Input: dimensioned drawing with shaded views. Units: mm. Origin: part minimum x, y, z. Coordinates: 2 decimals unless noted, no trailing zeros. Loops run counter-clockwise (first coordinate to the right, second up) from the corner with the lowest first, then second, coordinate; pieces in that order, holes last.
(1) Section C-C, the plane x = 20. Return loops of the section in (y, z), then the cut area to 3 significant figures.
(2) Section B-B, the plane z = 6. Return loops of the section in (x, y), then the cut area to 3 significant figures.
(3) Section A-A, the plane y = 8. Return loops of the section in (x, z), then the cut area to 3 significant figures.
(4) Contact query for a flat-ended pin moving along its axis: P1, Ø1.5, axis at x = 35.5, z = 6, coming from the -Y side. Output: stop coordinate, or through.
(5) Line query: L1, parallel to X at y = 2.25, z = 6; L2, parallel to Y at x = 20, z = 11.25; L3, parallel to X at y = 4, z = 4.75. Output: solid intervals per line, ascending.
(6) Section D-D, the plane y = 1.5. Return loops of the section in (x, z), then the cut area to 3 significant figures.
(7) Mould query, pull axis X, two halves, no side actions, for the marked faces 1, 2 and 3. Classes: released by +X, released by -X, zero draft, split by the parting line, or undercut.
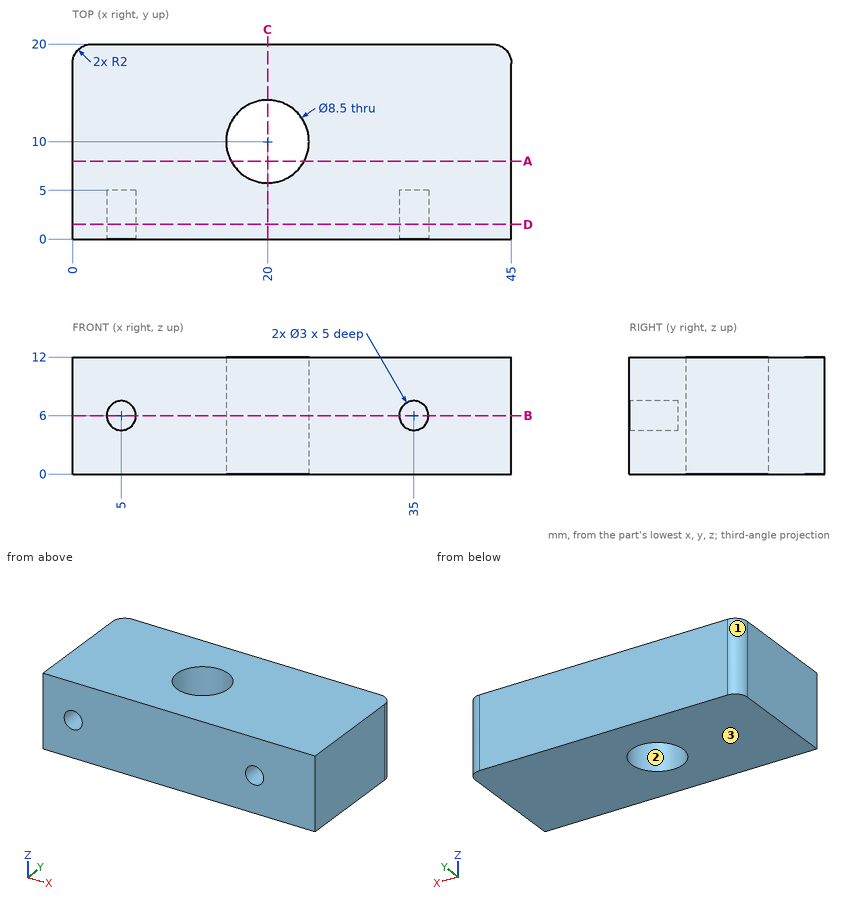
Report:
1. outline: (0, 0) - (5.75, 0) - (5.75, 12) - (0, 12) - close; (14.25, 0) - (20, 0) - (20, 12) - (14.25, 12) - close
1. area: 138 mm2
2. outline: (0, 0) - (3.5, 0) - (3.5, 5) - (6.5, 5) - (6.5, 0) - (33.5, 0) - (33.5, 5) - (36.5, 5) - (36.5, 0) - (45, 0) - (45, 18) arc R2 ccw to (43, 20) - (2, 20) arc R2 ccw to (0, 18) - close; hole circle Ø8.5 at (20, 10)
2. area: 812 mm2
3. outline: (0, 0) - (16.25, 0) - (16.25, 12) - (0, 12) - close; (23.75, 0) - (45, 0) - (45, 12) - (23.75, 12) - close
3. area: 450 mm2
4. P1: stops at y = 5
5. L1: x = 0 to 3.5, 6.5 to 33.5, 36.5 to 45
5. L2: y = 0 to 5.75, 14.25 to 20
5. L3: x = 0 to 4.17, 5.83 to 34.17, 35.83 to 45
6. outline: (0, 0) - (45, 0) - (45, 12) - (0, 12) - close; hole circle Ø3 at (5, 6); hole circle Ø3 at (35, 6)
6. area: 526 mm2
7. face 1: released by -X
7. face 2: undercut
7. face 3: zero draft
